Check sheet for the modelled part. Datum: model origin and axes. Units: mm. Face numbers are marked on the shaded views. A direction names the side the tool comes from. Give positions to 0.01 mm unless a question says otherwise; leave off trailing zeros. Order: outer loops, then holes, each group sorted by start corner. A loop starts at its lowest first (then second) coordinate and runs counter-clockwise, first axis right, second up.
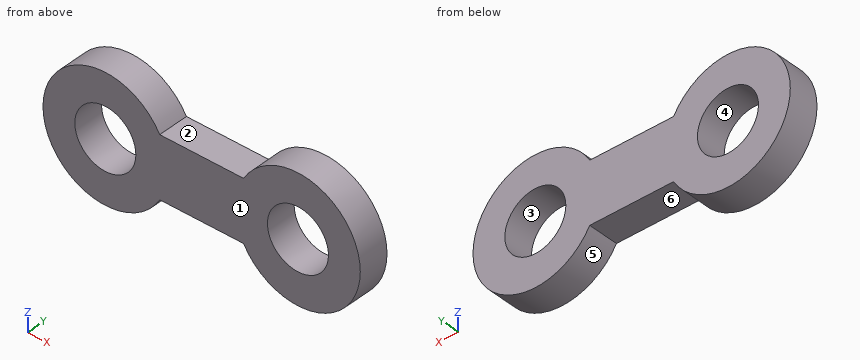
```python
from build123d import *

# Parameters (mm, degrees)
SKETCH4_R           = 40.863144044
SKETCH4_W           = 55
SKETCH4_H           = 40
BOSS_EXTRUDE1_DEPTH = 20
CUT_EXTRUDE1_REACH  = 115.513
SKETCH6_R           = 20


with BuildPart() as part:
    # Sketch4 → Boss-Extrude1 (new body)
    with BuildSketch(Plane(origin=(0, 0, 0), x_dir=(1, 0, 0), z_dir=(0, 1, 0))):
        with Locations((-63.134204652, 0)):
            Circle(SKETCH4_R)
        with Locations((63.134204652, 0)):
            Circle(SKETCH4_R)
        Rectangle(SKETCH4_W, SKETCH4_H)
    extrude(amount=BOSS_EXTRUDE1_DEPTH)

    # Sketch6 → Cut-Extrude1 (cut, up to next)
    with BuildSketch(Plane.XZ, mode=Mode.PRIVATE) as cut_extrude1_sk1:
        with Locations(Location((-63.134204652, 0, 0), (0, 0, 270))):
            Circle(SKETCH6_R)
    cut_extrude1_tool1 = extrude(cut_extrude1_sk1.sketch, amount=-CUT_EXTRUDE1_REACH, mode=Mode.PRIVATE) & part.part
    # Sketch6 → Cut-Extrude1 (cut, up to next)
    with BuildSketch(Plane.XZ, mode=Mode.PRIVATE) as cut_extrude1_sk2:
        with Locations(Location((63.134204652, 0, 0), (0, 0, 270))):
            Circle(SKETCH6_R)
    cut_extrude1_tool2 = extrude(cut_extrude1_sk2.sketch, amount=-CUT_EXTRUDE1_REACH, mode=Mode.PRIVATE) & part.part
    add(cut_extrude1_tool1.solids().sort_by_distance((-63.134205, 0, 0))[0], mode=Mode.SUBTRACT)
    add(cut_extrude1_tool2.solids().sort_by_distance((63.134205, 0, 0))[0], mode=Mode.SUBTRACT)


solid = part.part
```
(1) Material ranges on L1, parallel to X at y = 8.25, z = 17.5; L2, parallel to Z at x = -63, y = 16.25; L3, parallel to X at y = 4.5, z = 2, recorded low to high.
Response values:
L1: x = -100.06 to -72.82, -53.45 to 53.45, 72.82 to 100.06
L2: z = -40.86 to -20, 20 to 40.86
L3: x = -103.95 to -83.03, -43.23 to 43.23, 83.03 to 103.95
(2) Gauge pin test, flat ends, axial feed: pin 1 Ø1 at (x, y) = (0, 11.5) entering from +Z; pin 2 Ø24 at (x, z) = (-63.13, 0) entering from +Y; pin 3 Ø2 at (x, y) = (-43.5, 9.5) entering from +Z; pin 4 Ø4 at (y, z) = (2.5, -31.5) entering from +X. Record the tip position at first contact, or that the pin passes through.
Response values:
pin 1: stops at z = 20
pin 2: passes through
pin 3: stops at z = 36.37
pin 4: stops at x = 91.41
(3) Set-up check for the marked faces 1 and 2: record each of +Z, -Z, +X, -X, +Y, -Y from which the full face is reachable in a straight line by a thin tool's end or side.
Response values:
face 1: +Z, -Z, +X, -X, -Y
face 2: +Z, +Y, -Y
(4) Cross-section at D-D on z = -16. Enter the section's corners in (x, y), then the cut area to 3 significant figures.
Response values:
outline: (-100.73, 0) - (-75.13, 0) - (-75.13, 20) - (-100.73, 20) - close; (-51.13, 0) - (51.13, 0) - (51.13, 20) - (-51.13, 20) - close; (75.13, 0) - (100.73, 0) - (100.73, 20) - (75.13, 20) - close
area: 3,070 mm2
(5) Cross-section at A-A on z = 0. Enter the section's corners in (x, y).
Response values:
outline: (-104, 0) - (-83.13, 0) - (-83.13, 20) - (-104, 20) - close; (-43.13, 0) - (43.13, 0) - (43.13, 20) - (-43.13, 20) - close; (83.13, 0) - (104, 0) - (104, 20) - (83.13, 20) - close
(6) Cross-section at C-C on y = 12.25. Enter the section's corners in (x, z).
Response values:
outline: (-27.5, -20) - (27.5, -20) arc R40.86 ccw (long way) to (27.5, 20) - (-27.5, 20) arc R40.86 ccw (long way) to start; hole circle Ø40 at (-63.13, 0); hole circle Ø40 at (63.13, 0)
(7) Release check for a two-part mould opening along Z. For the marked faces 3, 4, 5 and 6 record: released by +Z, released by -Z, zero draft, split by the parting line, or undercut.
Response values:
face 3: undercut
face 4: undercut
face 5: split by the parting line
face 6: released by -Z
(8) Cross-section at B-B on x = -68. Enter the section's corners in (y, z).
Response values:
outline: (0, -40.57) - (20, -40.57) - (20, -19.4) - (0, -19.4) - close; (0, 19.4) - (20, 19.4) - (20, 40.57) - (0, 40.57) - close
